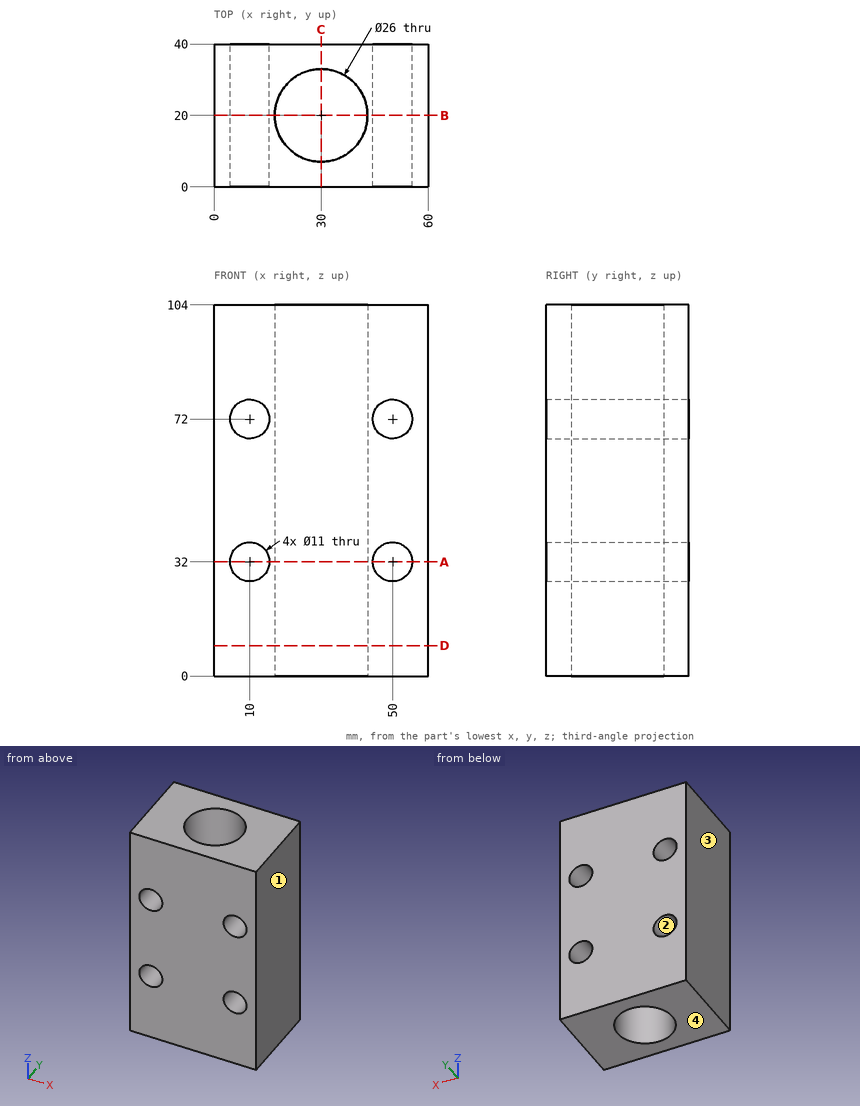
Verification items for this drawing (mm, ordinates from the low corner). Give positions to 0.01 mm unless a question says otherwise; leave off trailing zeros. Write each loop counter-clockwise with the first axis right and the second up, starting at its lowest first coordinate (ties: lowest second). Pieces come first, ordered by that corner, then holes. Notation, with made-up numbers: (56, 6.5) -> (76, 6.5) arc R16 ccw to (76, 13.5) -> close; hole circle Ø5 at (46, 25.5). An arc over 180 degrees is marked (long way). Use one line per item in the form item = value.
Item 1: Mould release check, pull along X, two halves, no side actions. Record for the marked faces 1, 2, 3 and 4: released by +X, released by -X, zero draft, split by the parting line, or undercut.
Results list:
face_1 = released by +X
face_2 = undercut
face_3 = released by -X
face_4 = zero draft
Item 2: Sectioned sample at D-D on z = 8.5. Enter the section's corners in (x, y).
Results list:
outline = (0, 0) -> (60, 0) -> (60, 40) -> (0, 40) -> close; hole circle Ø26 at (30, 20)
Item 3: Scan lines: line 1 (Z direction, x = 50, y = 29); line 2 (Z direction, x = 54.5, y = 34); line 3 (X direction, y = 20, z = 27). Record each from-to range of solid material in increasing order.
Results list:
line_1 = 0 to 26.5, 37.5 to 66.5, 77.5 to 104
line_2 = 0 to 28.84, 35.16 to 68.84, 75.16 to 104
line_3 = 0 to 7.71, 12.29 to 17, 43 to 47.71, 52.29 to 60
Item 4: Sectioned sample at C-C on x = 30. Enter the section's corners in (y, z).
Results list:
outline = (0, 0) -> (7, 0) -> (7, 104) -> (0, 104) -> close; (33, 0) -> (40, 0) -> (40, 104) -> (33, 104) -> close
Item 5: Sectioned sample at B-B on y = 20. Enter the section's corners in (x, z), plus the area to 3 significant figures.
Results list:
outline = (0, 0) -> (17, 0) -> (17, 104) -> (0, 104) -> close; (43, 0) -> (60, 0) -> (60, 104) -> (43, 104) -> close; hole circle Ø11 at (10, 32); hole circle Ø11 at (10, 72); hole circle Ø11 at (50, 32); hole circle Ø11 at (50, 72)
area = 3,160 mm2
Item 6: Sectioned sample at A-A on z = 32. Enter the section's corners in (x, y), plus the area to 3 significant figures.
Results list:
outline = (0, 0) -> (4.5, 0) -> (4.5, 40) -> (0, 40) -> close; (15.5, 0) -> (44.5, 0) -> (44.5, 40) -> (15.5, 40) -> close; (55.5, 0) -> (60, 0) -> (60, 40) -> (55.5, 40) -> close; hole circle Ø26 at (30, 20)
area = 989 mm2
